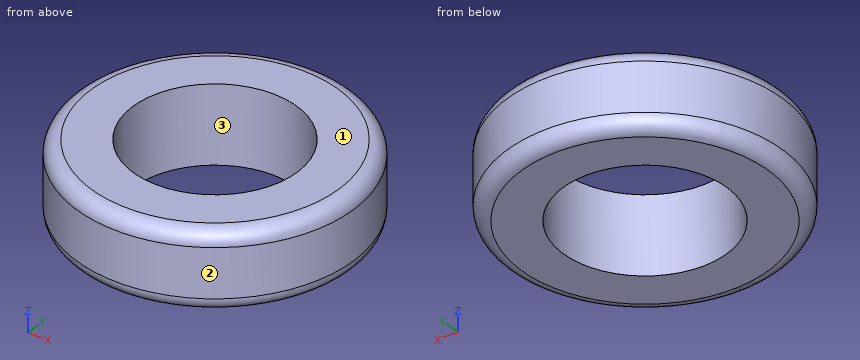
```python
from build123d import *

# Parameters (mm, degrees)
SKETCH_3_R          = 96.5
EXTRUDE_1_DEPTH     = 54.23
FILLET_1_R          = 10
SKETCH_4_R          = 57.34
CUT_EXTRUDE_1_DEPTH = 54.23


with BuildPart() as part:
    # 草图3 → 凸台-拉伸1 (new body)
    with BuildSketch(Plane.XY):
        with Locations((58.742605219, 48.942624637)):
            Circle(SKETCH_3_R)
    extrude(amount=EXTRUDE_1_DEPTH)

    # 圆角1
    fillet_1_edges = [part.edges().sort_by_distance(p)[0] for p in [
        (-37.757394781, 48.942624637, 0),
        (-37.757394781, 48.942624637, 54.23),
    ]]
    fillet(fillet_1_edges, radius=FILLET_1_R)

    # 草图4 → 切除-拉伸1 (cut)
    with BuildSketch(Plane.XY.offset(54.23)):
        with Locations((58.742605219, 48.942624637)):
            Circle(SKETCH_4_R)
    extrude(amount=-CUT_EXTRUDE_1_DEPTH, mode=Mode.SUBTRACT)


solid = part.part
```
Here's how the part is built. I have some questions about the finished solid (model axes, mm). Face numbers are marked on the shaded views. Give positions to 0.01 mm unless a question says otherwise; leave off trailing zeros. Write each loop counter-clockwise with the first axis right and the second up, starting at its lowest first coordinate (ties: lowest second). Pieces come first, ordered by that corner, then holes. Notation, with made-up numbers: M 80.5,25.5 L 102.5,25.5 A28 cw 102.5,63.5 Z; hole C -11.75,83 d4. An arc over 180 degrees is marked long. Put each result on its own line as item: value. Start each with the question number.
Item 1: I need wall thicknesses on L1, parallel to X at y = 48, z = 12; L2, parallel to X at y = 82.5, z = 28.5; L3, parallel to Y at x = 106.5, z = 16. Which ranges of each line are inside material? Lowest first, please. Write a range as from..to.
Item 2: If we section it at B-B, the plane z = 6.5: Write out the boundary of the cut face in (x, y) (1 decimal), then the cut area to 3 significant figures.
Item 3: Will these pins go through, and if not, where does the flat tip stop? pin 1 (10 mm diameter, centred on x = 45, z = 46, fed in from +Y); pin 2 (3 mm diameter, centred on x = 106, z = 31, fed in from +Y); pin 3 (8 mm diameter, centred on x = 91, z = 45, fed in from +Y).
Item 4: If we section it at A-A, the plane z = 30: Write out the boundary of the cut face in (x, y), then the cut area to 3 significant figures.
Item 5: Thinking about a two-plate mould opening in X: for the marked faces 1, 2 and 3, which applies, +X half, -X half, draft (parallel to the pull), parting line (faces both ways), or undercut?
Values:
1. L1: -37.75..1.41, 116.07..155.24
1. L2: -31.73..12.25, 105.24..149.22
1. L3: -34.91..17.21, 80.68..132.8
2. outline: C 58.7,48.9 d191.7; hole C 58.7,48.9 d114.7
2. area: 18,500 mm²
3. pin 1: y = 145.02
3. pin 2: y = 133.9
3. pin 3: y = 141.2
4. outline: C 58.74,48.94 d193; hole C 58.74,48.94 d114.68
4. area: 18,900 mm²
5. face 1: draft
5. face 2: parting line
5. face 3: undercut
